The listing builds one solid part. Answer for the finished solid, in the listing's coordinates (mm). A direction names the side the tool comes from. Round coordinates to 2 decimals unless told otherwise and drop trailing zeros. Write each loop counter-clockwise with the first axis right and the second up, starting at its lowest first coordinate (ties: lowest second). Pieces come first, ordered by that corner, then holes.
Item 1: For a pull along X with two mould halves and no side action, classify faces 3 (the face through (0.2, 12.3, 24.5)), 4 (the face through (-12.5, 12, 25)), 5 (the face through (13.164, 12.325, 16.26)) as +X half, -X half, draft (parallel to the pull), parting line (faces both ways), or undercut.
Item 2: Find the intervals of material crossed by probe 1 along X at (y, z) = (20.5, 21); probe 2 along X at (y, z) = (10.5, 5.5); probe 3 along X at (y, z) = (3, 3.5), in increasing order.
Item 3: A tool of negligible diameter and unlimited length cuts with its end or side. For faces 1 (the face through (0, 25, 15)), 2 (the face through (12.5, 12, 25)), from which of +Z, -Z, +X, -X, +Y, -Y can it reach the whole face along a straight path? Write none if from no direction.
Item 4: Find section D-D on z = 25.5. Give the vertices of the cut face in (x, y).
Item 5: Find section A-A on z = 12. Give the vertices of the cut face in (x, y), then the cut area to 3 significant figures.
Item 6: Find section C-C on x = 0. Give the vertices of the cut face in (y, z).
Item 7: Each of these flat-tipped pins is pushed along its axis until it touches: pin 1 (3 mm diameter, centred on y = 13, z = 23.5, fed in from -X); pin 2 (2 mm diameter, centred on y = 17.5, z = 25, fed in from +X); pin 3 (10 mm diameter, centred on y = 21.5, z = 9.5, fed in from -X). Where does it stop, or does it pass through?
Item 8: Find section B-B on y = 19.5. Give the vertices of the cut face in (x, z).
```python
from build123d import *

# Parameters (mm, degrees)
EXTRUDE_1_DEPTH     = 25
SKETCH_2_W          = 28.626473145
SKETCH_2_H          = 10
CUT_EXTRUDE_1_DEPTH = 49.928519291


with BuildPart() as part:
    # Эскиз1 → Бобышка-Вытянуть1 (new body)
    with BuildSketch(Plane(origin=(0, 0, 0), x_dir=(1, 0, 0), z_dir=(0, 1, 0))):
        with BuildLine():
            Line((-12.5, -37), (-12.5, -19.843134833))
            ThreePointArc((-12.5, -19.843134833), (-13.145856533, -16.307600927), (-15, -13.228756555))
            ThreePointArc((-15, -13.228756555), (-18.708286934, -7.071067812), (-20, 0))
            Line((-20, 0), (-13.5, 0))
            ThreePointArc((-13.5, 0), (0, -13.5), (13.5, 0))
            Line((13.5, 0), (20, 0))
            ThreePointArc((20, 0), (18.708286934, -7.071067812), (15, -13.228756555))
            ThreePointArc((15, -13.228756555), (13.145856533, -16.307600927), (12.5, -19.843134833))
            Line((12.5, -19.843134833), (12.5, -37))
            ThreePointArc((12.5, -37), (0, -24.5), (-12.5, -37))
        make_face()
    extrude(amount=EXTRUDE_1_DEPTH)

    # Эскиз2 → Вырез-Вытянуть1 (cut, through all)
    with BuildSketch(Plane(origin=(0, 25, 0), x_dir=(1, 0, 0), z_dir=(0, 1, 0))):
        with Locations((0.56499618, -35.5)):
            Rectangle(SKETCH_2_W, SKETCH_2_H)
    extrude(amount=-CUT_EXTRUDE_1_DEPTH, mode=Mode.SUBTRACT)


solid = part.part
```
Check values:
1. face 3: undercut
1. face 4: -X half
1. face 5: +X half
2. probe 1: x = -12.5 to 12.5
2. probe 2: x = -19.23 to -12.33, 12.33 to 19.23
2. probe 3: x = -19.69 to -13.04, 13.04 to 19.69
3. face 1: +Z, -Z, +X, -X, +Y
3. face 2: +Z, +X, +Y, -Y
4. outline: (-12.5, 0) - (-4.9, 0) - (-4.9, 25) - (-12.5, 25) - close; (4.9, 0) - (12.5, 0) - (12.5, 25) - (4.9, 25) - close
5. outline: (-16, 0) - (-6.18, 0) - (-6.18, 25) - (-16, 25) - close; (6.18, 0) - (16, 0) - (16, 25) - (6.18, 25) - close
5. area: 491 mm2
6. outline: (0, 13.5) - (25, 13.5) - (25, 24.5) - (0, 24.5) - close
7. pin 1: stops at x = -12.5
7. pin 2: stops at x = 12.5
7. pin 3: stops at x = -19.49
8. outline: (-20, 0) - (-13.5, 0) arc R13.5 cw to (13.5, 0) - (20, 0) arc R20 ccw to (15, 13.23) arc R10 cw to (12.5, 19.84) - (12.5, 30.5) - (10.68, 30.5) arc R12.5 cw to (-10.68, 30.5) - (-12.5, 30.5) - (-12.5, 19.84) arc R10 cw to (-15, 13.23) arc R20 ccw to start
